Design review of the part built by this model. Coordinates are the model's own, in mm. A direction names the side the tool comes from. Round coordinates to 2 decimals unless told otherwise and drop trailing zeros. Loops run counter-clockwise (first coordinate to the right, second up) from the corner with the lowest first, then second, coordinate; pieces in that order, holes last. Notation, with made-up numbers: (-30.75, 10) - (15.25, 10) arc R11 ccw to (15.25, 28) - close; hole circle Ø5 at (-20, 49). An arc over 180 degrees is marked (long way). Return JSON: item names as keys, results as strings. Group by question number.
(1) We need section B-B, the plane x = 12.5. Write out the cut boundary in (y, z).
(2) Clearance check with flat-ended pins moving along their axes: pin 1 (1.1 mm diameter, centred on y = 6, z = 1.5, fed in from -X); pin 2 (1 mm diameter, centred on x = 10.5, y = -4, fed in from +Z); pin 3 (5 mm diameter, centred on x = 15, z = 7.5, fed in from +Y). State where each tip first meets the part, or that it passes through.
(3) We need section D-D, the plane z = 2.5. Write out the cut boundary in (x, y).
(4) We need section A-A, the plane y = 3.5. Write out the cut boundary in (x, z), and give its area (3 significant figures).
(5) The part is to be moulded in two halves that separate along Z. For faces 4 (the flat face through (13, 3, 7)), 5 (the cylindrical face through (9.1, -2.7, -3.3)), 6 (the flat face through (13, 9, -1)), say which applies: pulls with the +Z half, pulls with the -Z half, needs draft (parallel to the pull), parting line crosses it, or undercut.
(6) For faces 1 (the flat face through (13, -3, 18.654)), 2 (the flat face through (16, 6, 12.833)), 3 (the flat face through (11, 6, 0.733)), list the 3-axis set-ups (+Z, -Z, +X, -X, +Y, -Y) from which the entire face can be reached by the end or side of a thin tool; tool diameter is ignored.
(7) Wall thickness on L1, parallel to Z at x = 14.25, y = 3.5; L2, parallel to Y at x = 13.75, z = 7.25; L3, parallel to Z at x = 9, y = 7.25: over which ranges is each line inside the solid? List them lowest first. Write a range as [from, to].
(8) We need section C-C, the plane y = -11.75. Write out the cut boundary in (x, z), and give its area (3 significant figures).
from build123d import *

# Parameters (mm, degrees)
CROQUIS1_R                 = 2.4
SALIENTE_EXTRUIR1_DEPTH    = 3
SALIENTE_EXTRUIR2_DEPTH    = 6
CORTAR_EXTRUIR4_DEPTH      = 48.064644057
CORTAR_EXTRUIR4_DEPTH_BACK = 3
SALIENTE_EXTRUIR3_START    = 14
SALIENTE_EXTRUIR3_DEPTH    = 14


with BuildPart() as part:
    # Croquis1 → Saliente-Extruir1 (new body)
    with BuildSketch(Plane(origin=(0, 0, 0), x_dir=(1, 0, 0), z_dir=(0, 1, 0))):
        with BuildLine():
            Line((35.117506554, -10.768616799), (17.851894103, -10.768616799))
            Line((17.851894103, -10.768616799), (17.851894103, -15.511473942))
            ThreePointArc((17.851894103, -15.511473942), (16.931372558, -17.73380954), (14.70903696, -18.654331085))
            Line((14.70903696, -18.654331085), (11.280465531, -18.654331085))
            ThreePointArc((11.280465531, -18.654331085), (9.058129933, -17.73380954), (8.137608389, -15.511473942))
            Line((8.137608389, -15.511473942), (8.137608389, 1.036415275))
            ThreePointArc((8.137608389, 1.036415275), (9.058129933, 3.258750873), (11.280465531, 4.179272418))
            Line((11.280465531, 4.179272418), (14.70903696, 4.179272418))
            ThreePointArc((14.70903696, 4.179272418), (16.931372558, 3.258750873), (17.851894103, 1.036415275))
            Line((17.851894103, 1.036415275), (17.851894103, -3.797188228))
            Line((17.851894103, -3.797188228), (35.117506554, -3.797188228))
            ThreePointArc((35.117506554, -3.797188228), (42.791315147, -7.282902513), (35.117506554, -10.768616799))
        make_face()
        with Locations(Location((38.162743718, -7.282902513, 0), (0, 0, 270))):
            Circle(CROQUIS1_R, mode=Mode.SUBTRACT)
    extrude(amount=SALIENTE_EXTRUIR1_DEPTH)

    # Croquis2 → Saliente-Extruir2 (add)
    with BuildSketch(Plane(origin=(0, 3, 0), x_dir=(1, 0, 0), z_dir=(0, 1, 0))):
        with BuildLine():
            Line((13.22040734, -0.732902513), (13.22040734, -1.732902513))
            Line((13.22040734, -1.732902513), (17.851894103, -1.732902513))
            Line((17.851894103, -1.732902513), (17.851894103, 1.036415275))
            ThreePointArc((17.851894103, 1.036415275), (16.931372558, 3.258750873), (14.70903696, 4.179272418))
            Line((14.70903696, 4.179272418), (11.280465531, 4.179272418))
            ThreePointArc((11.280465531, 4.179272418), (9.058129933, 3.258750873), (8.137608389, 1.036415275))
            Line((8.137608389, 1.036415275), (8.137608389, -0.732902513))
            Line((8.137608389, -0.732902513), (13.22040734, -0.732902513))
        make_face()
        with BuildLine():
            Line((17.851894103, -12.832902513), (13.22040734, -12.832902513))
            Line((13.22040734, -12.832902513), (13.22040734, -13.832902513))
            Line((13.22040734, -13.832902513), (8.137608389, -13.832902513))
            Line((8.137608389, -13.832902513), (8.137608389, -15.511473942))
            ThreePointArc((8.137608389, -15.511473942), (9.058129933, -17.73380954), (11.280465531, -18.654331085))
            Line((11.280465531, -18.654331085), (14.70903696, -18.654331085))
            ThreePointArc((14.70903696, -18.654331085), (16.931372558, -17.73380954), (17.851894103, -15.511473942))
            Line((17.851894103, -15.511473942), (17.851894103, -12.832902513))
        make_face()
    extrude(amount=SALIENTE_EXTRUIR2_DEPTH)

    # Croquis3 → Cortar-Extruir4 (cut, two sides: drawn at the far end of the back side and taken through both)
    with BuildSketch(Plane(origin=(0, 3, 0), x_dir=(1, 0, 0), z_dir=(0, 1, 0)).offset(-CORTAR_EXTRUIR4_DEPTH_BACK)):
        Polygon((17.851894103, 64.354823399), (17.851894103, -3.797188228), (17.851894103, -10.768616799), (17.851894103, -78.920628426), (154.155917357, -78.920628426), (154.155917357, 64.354823399), align=None)
    extrude(amount=CORTAR_EXTRUIR4_DEPTH + CORTAR_EXTRUIR4_DEPTH_BACK, mode=Mode.SUBTRACT)

    # Croquis4 → Saliente-Extruir3 (add)
    with BuildSketch(Plane.XZ.offset(SALIENTE_EXTRUIR3_START)):
        with BuildLine():
            Line((17.851894103, 15.511473942), (17.851894103, -1.036415275))
            ThreePointArc((17.851894103, -1.036415275), (16.931372558, -3.258750873), (14.70903696, -4.179272418))
            Line((14.70903696, -4.179272418), (11.280465531, -4.179272418))
            ThreePointArc((11.280465531, -4.179272418), (9.058129933, -3.258750873), (8.137608389, -1.036415275))
            Line((8.137608389, -1.036415275), (8.137608389, 15.511473942))
            ThreePointArc((8.137608389, 15.511473942), (9.058129933, 17.73380954), (11.280465531, 18.654331085))
            Line((11.280465531, 18.654331085), (14.70903696, 18.654331085))
            ThreePointArc((14.70903696, 18.654331085), (16.931372558, 17.73380954), (17.851894103, 15.511473942))
        make_face()
    extrude(amount=-SALIENTE_EXTRUIR3_DEPTH)


solid = part.part
Solutions:
{
 "1": {"outline": "(-14, -4.18) - (9, -4.18) - (9, 0.73) - (3, 0.73) - (3, 13.83) - (9, 13.83) - (9, 18.65) - (-14, 18.65) - close"},
 "2": {"pin 1": "x = 13.22", "pin 2": "z = 18.64", "pin 3": "y = 3"},
 "3": {"outline": "(8.14, -14) - (17.85, -14) - (17.85, 3) - (8.14, 3) - close"},
 "4": {"outline": "(8.14, -1.04) arc R3.14 ccw to (11.28, -4.18) - (14.71, -4.18) arc R3.14 ccw to (17.85, -1.04) - (17.85, 1.73) - (13.22, 1.73) - (13.22, 0.73) - (8.14, 0.73) - close; (8.14, 13.83) - (13.22, 13.83) - (13.22, 12.83) - (17.85, 12.83) - (17.85, 15.51) arc R3.14 ccw to (14.71, 18.65) - (11.28, 18.65) arc R3.14 ccw to (8.14, 15.51) - close", "area": "95.3 mm^2"},
 "5": {"face 4": "undercut", "face 5": "pulls with the -Z half", "face 6": "needs draft"},
 "6": {"face 1": "+Z, +X, -X, +Y, -Y", "face 2": "+X, -X, +Y", "face 3": "-X, +Y"},
 "7": {"L1": "[-4.18, 1.73], [12.83, 18.65]", "L2": "[-14, 3]", "L3": "[-3.2, 0.73], [13.83, 17.67]"},
 "8": {"outline": "(8.14, -1.04) arc R3.14 ccw to (11.28, -4.18) - (14.71, -4.18) arc R3.14 ccw to (17.85, -1.04) - (17.85, 15.51) arc R3.14 ccw to (14.71, 18.65) - (11.28, 18.65) arc R3.14 ccw to (8.14, 15.51) - close", "area": "213 mm^2"}
}
